The listing builds one solid part. Answer for the finished solid, in the listing's coordinates (mm). Coordinates: 2 decimals unless noted, no trailing zeros. Order: outer loops, then holes, each group sorted by start corner. A loop starts at its lowest first (then second) coordinate and runs counter-clockwise, first axis right, second up. Notation, with made-up numbers: (27.25, 16) -> (49.25, 16) arc R4 cw to (49.25, 23) -> close; hole circle Ø3 at (84, 67). An arc over 180 degrees is marked (long way). Put each result on its own line as item: value. Start each with the question number.
```python
from build123d import *

# Parameters (mm, degrees)
SKETCH1_R           = 4.354315493
BOSS_EXTRUDE1_DEPTH = 12.7
CUT_EXTRUDE1_DEPTH  = 25.4
CUT_EXTRUDE2_DEPTH  = 25.4


with BuildPart() as part:
    # Sketch1 → Boss-Extrude1 (new body)
    with BuildSketch(Plane.XY):
        with BuildLine():
            ThreePointArc((-3.792038647, 8.146354139), (-8.146354139, 3.792038647), (-12.500669632, 8.146354139))
            Line((-12.500669632, 8.146354139), (-12.500669632, -8.146354139))
            ThreePointArc((-12.500669632, -8.146354139), (-8.146354139, -3.792038647), (-3.792038647, -8.146354139))
            ThreePointArc((-3.792038647, -8.146354139), (-5.067388127, -11.225320151), (-8.146354139, -12.500669632))
            Line((-8.146354139, -12.500669632), (8.146354139, -12.500669632))
            ThreePointArc((8.146354139, -12.500669632), (5.067388127, -5.067388127), (12.500669632, -8.146354139))
            Line((12.500669632, -8.146354139), (12.500669632, 8.146354139))
            ThreePointArc((12.500669632, 8.146354139), (5.067388127, 5.067388127), (8.146354139, 12.500669632))
            Line((8.146354139, 12.500669632), (-8.146354139, 12.500669632))
            ThreePointArc((-8.146354139, 12.500669632), (-5.067388127, 11.225320151), (-3.792038647, 8.146354139))
        make_face()
        with Locations((-8.146354139, 8.146354139)):
            Circle(SKETCH1_R)
        with Locations((-8.146354139, -8.146354139)):
            Circle(SKETCH1_R)
        with Locations((8.146354139, 8.146354139)):
            Circle(SKETCH1_R)
        with Locations((8.146354139, -8.146354139)):
            Circle(SKETCH1_R)
    extrude(amount=BOSS_EXTRUDE1_DEPTH)

    # Sketch2 → Cut-Extrude1 (cut, symmetric)
    with BuildSketch(Plane(origin=(0, 0, 0), x_dir=(0, 0, -1), z_dir=(1, 0, 0))):
        Polygon((-12.7, 12.500669632), (-1.5875, 12.500669632), (-12.7, 8.456050403), align=None)
        Polygon((-1.5875, -12.500669632), (-12.7, -8.456050403), (-12.7, -12.500669632), align=None)
    extrude(amount=CUT_EXTRUDE1_DEPTH, both=True, mode=Mode.SUBTRACT)

    # Sketch3 → Cut-Extrude2 (cut, symmetric)
    with BuildSketch(Plane(origin=(0, 0, 0), x_dir=(1, 0, 0), z_dir=(0, 1, 0))):
        Polygon((12.500669632, -1.5875), (8.456050403, -12.7), (12.500669632, -12.7), align=None)
        Polygon((-8.456050403, -12.7), (-12.500669632, -12.7), (-12.500669632, -1.5875), align=None)
    extrude(amount=CUT_EXTRUDE2_DEPTH, both=True, mode=Mode.SUBTRACT)


solid = part.part
```
(1) The part is cut by section B-B on z = 4.5. Determine the outline of the cut face in (x, y), plus the area to 3 significant figures.
(2) The part is cut by section A-A on x = -3. Determine the outline of the cut face in (y, z), plus the area to 3 significant figures.
(3) Each of these flat-tipped pins is pushed along its axis until it touches: P1, Ø3, axis at x = 1.5, y = -5.5, coming from the -Z side; P2, Ø1, axis at x = -2, z = 9, coming from the +Y side; P3, Ø1, axis at y = 8, z = 4.5, coming from the -X side; P4, Ø6, axis at x = -1.5, z = 5.5, coming from the -Y side. Where does it stop, or does it pass through?
(4) The part is cut by section D-D on z = 2.75. Determine the outline of the cut face in (x, y), plus the area to 3 significant figures.
(5) Find the intervals of material crossed by L1, parallel to X at y = 7.25, z = 6.5; L2, parallel to Y at x = 4.75, z = 7.75; L3, parallel to X at y = 1, z = 6, in increasing order.
Worked out:
1. outline: (-11.44, -10.99) arc R4.35 ccw to (-10.99, -11.44) -> (10.99, -11.44) arc R4.35 ccw to (11.44, -10.99) -> (11.44, 10.99) arc R4.35 ccw to (10.99, 11.44) -> (-10.99, 11.44) arc R4.35 ccw to (-11.44, 10.99) -> close
1. area: 523 mm2
2. outline: (-12.5, 0) -> (12.5, 0) -> (12.5, 1.59) -> (8.46, 12.7) -> (-8.46, 12.7) -> (-12.5, 1.59) -> close
2. area: 273 mm2
3. P1: z = 0
3. P2: y = 9.98
3. P3: x = -11.62
3. P4: y = -12.17
4. outline: (-12.08, -10.02) arc R4.35 ccw to (-10.02, -12.08) -> (10.02, -12.08) arc R4.35 ccw to (12.08, -10.02) -> (12.08, 10.02) arc R4.35 ccw to (10.02, 12.08) -> (-10.02, 12.08) arc R4.35 ccw to (-12.08, 10.02) -> close
4. area: 577 mm2
5. L1: -10.71 to 10.71
5. L2: -10.26 to 10.26
5. L3: -10.89 to 10.89
